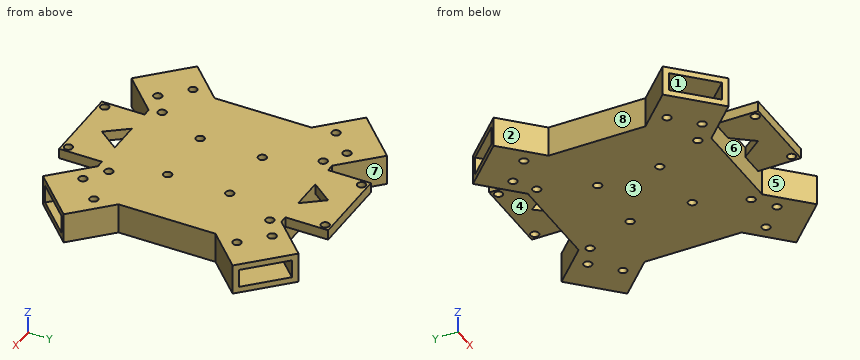
```python
from build123d import *

# Parameters (mm, degrees)
SKETCH1_W           = 90
SKETCH1_H           = 90
SKETCH1_R           = 2.05
BOSS_EXTRUDE1_DEPTH = 15
BOSS_EXTRUDE2_DEPTH = 15
SKETCH4_R           = 2.05
CUT_EXTRUDE1_DEPTH  = 15
SKETCH6_W           = 24
SKETCH6_H           = 9.009591428
CUT_EXTRUDE2_DEPTH  = 22
SKETCH9_W           = 24
SKETCH9_H           = 9
CUT_EXTRUDE3_DEPTH  = 22
SKETCH7_W           = 24
SKETCH7_H           = 9
CUT_EXTRUDE4_DEPTH  = 22
SKETCH8_W           = 24
SKETCH8_H           = 9
CUT_EXTRUDE5_DEPTH  = 22
SKETCH10_R          = 2.05
BOSS_EXTRUDE3_DEPTH = 5


with BuildPart() as part:
    # Sketch1 → Boss-Extrude1 (new body)
    with BuildSketch(Plane(origin=(0, 0, 0), x_dir=(0, 1, 0), z_dir=(0, 0, 1))):
        with Locations((-1.369565217, -20.064677945)):
            Rectangle(SKETCH1_W, SKETCH1_H)
        with Locations(Location((-40.369565217, 4.935322055, 0), (0, 0, 270))):
            Circle(SKETCH1_R, mode=Mode.SUBTRACT)
        with Locations(Location((-40.369565217, -45.064677945, 0), (0, 0, 270))):
            Circle(SKETCH1_R, mode=Mode.SUBTRACT)
        with Locations(Location((38.630434783, 4.935322055, 0), (0, 0, 270))):
            Circle(SKETCH1_R, mode=Mode.SUBTRACT)
        with Locations(Location((38.630434783, -45.064677945, 0), (0, 0, 270))):
            Circle(SKETCH1_R, mode=Mode.SUBTRACT)
        with Locations(Location((13.880434783, -4.814677945, 0), (0, 0, 270))):
            Circle(SKETCH1_R, mode=Mode.SUBTRACT)
        with Locations(Location((-16.619565217, -4.814677945, 0), (0, 0, 270))):
            Circle(SKETCH1_R, mode=Mode.SUBTRACT)
        with Locations(Location((13.880434783, -35.314677945, 0), (0, 0, 270))):
            Circle(SKETCH1_R, mode=Mode.SUBTRACT)
        with Locations(Location((-16.619565217, -35.314677945, 0), (0, 0, 270))):
            Circle(SKETCH1_R, mode=Mode.SUBTRACT)
    extrude(amount=BOSS_EXTRUDE1_DEPTH)

    # Sketch2 → Boss-Extrude2 (add)
    with BuildSketch(Plane.XY.offset(15)):
        Polygon((-21.399788149, 61.308104312), (-42.612991584, 40.094900877), (-24.935322055, 22.417231347), (-24.935322055, 43.630434783), (-3.722118619, 43.630434783), align=None)
        Polygon((-24.935322055, -25.156361782), (-42.612991584, -42.834031311), (-21.399788149, -64.047234747), (-3.722118619, -46.369565217), (-24.935322055, -46.369565217), align=None)
        Polygon((61.529144039, 61.308104312), (43.85147451, 43.630434783), (65.064677945, 43.630434783), (65.064677945, 22.417231347), (82.742347475, 40.094900877), align=None)
        Polygon((43.85147451, -46.369565217), (61.529144039, -64.047234747), (82.742347475, -42.834031311), (65.064677945, -25.156361782), (65.064677945, -46.369565217), align=None)
    extrude(amount=-BOSS_EXTRUDE2_DEPTH)

    # Sketch4 → Cut-Extrude1 (cut)
    with BuildSketch(Plane.XY.offset(15)):
        with Locations((-26.349535617, 33.730939846)):
            Circle(SKETCH4_R)
        with Locations((-15.035827118, 45.044648345)):
            Circle(SKETCH4_R)
        with Locations(Location((66.478891508, 33.730939846, 0), (0, 0, 180))):
            Circle(SKETCH4_R)
        with Locations(Location((55.165183009, 45.044648345, 0), (0, 0, 180))):
            Circle(SKETCH4_R)
        with Locations((66.478891508, -36.470070281)):
            Circle(SKETCH4_R)
        with Locations((55.165183009, -47.78377878)):
            Circle(SKETCH4_R)
        with Locations(Location((-15.035827118, -47.78377878, 0), (0, 0, 180))):
            Circle(SKETCH4_R)
        with Locations(Location((-26.349535617, -36.470070281, 0), (0, 0, 180))):
            Circle(SKETCH4_R)
    extrude(amount=-CUT_EXTRUDE1_DEPTH, mode=Mode.SUBTRACT)

    # Sketch6 → Cut-Extrude2 (cut)
    with BuildSketch(Plane(origin=(-41.35394623, 41.35394623, 0), x_dir=(-0.7071067811865476, -0.7071067811865476, 0), z_dir=(-0.7071067811865476, 0.7071067811865476, 0))):
        with Locations((-13.219440985, 7.504795714)):
            Rectangle(SKETCH6_W, SKETCH6_H)
    extrude(amount=-CUT_EXTRUDE2_DEPTH, mode=Mode.SUBTRACT)

    # Sketch9 → Cut-Extrude3 (cut)
    with BuildSketch(Plane(origin=(61.418624176, 61.418624176, 0), x_dir=(-0.7071067811865479, 0.7071067811865472, 0), z_dir=(0.7071067811865472, 0.7071067811865479, 0))):
        with Locations((-15.15629869, 7.5)):
            Rectangle(SKETCH9_W, SKETCH9_H)
    extrude(amount=-CUT_EXTRUDE3_DEPTH, mode=Mode.SUBTRACT)

    # Sketch7 → Cut-Extrude4 (cut)
    with BuildSketch(Plane(origin=(-42.723511448, -42.723511448, 0), x_dir=(0.7071067811865483, -0.7071067811865468, 0), z_dir=(-0.7071067811865468, -0.7071067811865483, 0))):
        with Locations((15.15629869, 7.5)):
            Rectangle(SKETCH7_W, SKETCH7_H)
    extrude(amount=-CUT_EXTRUDE4_DEPTH, mode=Mode.SUBTRACT)

    # Sketch8 → Cut-Extrude5 (cut)
    with BuildSketch(Plane(origin=(62.788189393, -62.788189393, 0), x_dir=(0.7071067811865461, 0.707106781186549, 0), z_dir=(0.707106781186549, -0.7071067811865461, 0))):
        with Locations((13.219440985, 7.5)):
            Rectangle(SKETCH8_W, SKETCH8_H)
    extrude(amount=-CUT_EXTRUDE5_DEPTH, mode=Mode.SUBTRACT)

    # Sketch10 → Boss-Extrude3 (add)
    # profile 1 of 2: a face of its own
    with BuildSketch(Plane.XY.offset(15)):
        Polygon((40.064677945, 64.630434783), (0.064677945, 64.630434783), (0.064677945, 43.630434783), (12.064677945, 43.630434783), (20.064677945, 54.130434783), (28.064677945, 43.630434783), (40.064677945, 43.630434783), align=None)
        with Locations((3.064677945, 61.630434783)):
            Circle(SKETCH10_R, mode=Mode.SUBTRACT)
        with Locations((37.064677945, 61.630434783)):
            Circle(SKETCH10_R, mode=Mode.SUBTRACT)
    # profile 2 of 2: a face of its own
    with BuildSketch(Plane.XY.offset(15)):
        Polygon((12.064677945, -46.369565217), (0.064677945, -46.369565217), (0.064677945, -67.369565217), (40.064677945, -67.369565217), (40.064677945, -46.369565217), (28.064677945, -46.369565217), (20.064677945, -56.869565217), align=None)
        with Locations((3.064677945, -64.369565217)):
            Circle(SKETCH10_R, mode=Mode.SUBTRACT)
        with Locations((37.064677945, -64.369565217)):
            Circle(SKETCH10_R, mode=Mode.SUBTRACT)
    extrude(amount=-BOSS_EXTRUDE3_DEPTH)


solid = part.part
```
CAD build for the part. Positions are in the model's coordinates, mm. Face numbers are marked on the shaded views. A direction names the side the tool comes from. Round coordinates to 2 decimals unless told otherwise and drop trailing zeros. Order: outer loops, then holes, each group sorted by start corner. A loop starts at its lowest first (then second) coordinate and runs counter-clockwise, first axis right, second up. Notation, with made-up numbers: (9, -25.75) -> (62, -25.75) arc R28 cw to (62, 1.25) -> close; hole circle Ø4 at (58.5, 72). An arc over 180 degrees is marked (long way). One line per question, with ' | ' between items.
Q1. Two-plate mould, pull along X, no slides. Class the marked faces 1, 2, 3 and 4: released by +X, released by -X, zero draft, split by the parting line, or undercut.
Completed:
face 1: undercut | face 2: released by -X | face 3: zero draft | face 4: undercut
Q2. Slice it at A-A (z = 1.5). Give the number of separate pieces and of enclosed holes in the cut face, then the cut area to 3 significant figures.
Completed:
separate pieces: 1 | enclosed holes: 16 | area: 9,990 mm^2
Q3. Drop flat-ended pins along their axis: pin 1 (2.5 mm diameter, centred on y = 58, z = 13.5, fed in from -X); pin 2 (1.5 mm diameter, centred on y = 58.5, z = 13, fed in from +X); pin 3 (6.5 mm diameter, centred on x = 35.31, y = -16.62, fed in from +Z); pin 4 (4 mm diameter, centred on y = -59.5, z = 12, fed in from +X). Give the stop position or say it passes through.
Completed:
pin 1: stops at x = -25.96 | pin 2: stops at x = 65.09 | pin 3: stops at z = 15 | pin 4: stops at x = 68.08
Q4. Slice it at B-B (y = 56.5). Write the cut outline in (x, z).
Completed:
outline: (-26.21, 0) -> (-16.59, 0) -> (-16.59, 15) -> (-26.21, 15) -> (-26.21, 12.01) -> (-20.83, 12.01) -> (-20.83, 3) -> (-26.21, 3) -> close; (0.06, 10) -> (40.06, 10) -> (40.06, 15) -> (0.06, 15) -> close; (56.72, 0) -> (66.34, 0) -> (66.34, 3) -> (60.96, 3) -> (60.96, 12) -> (66.34, 12) -> (66.34, 15) -> (56.72, 15) -> close
Q5. Slice it at C-C (x = 70.5). Write the cut outline in (y, z), then the cut area to 3 significant figures.
Completed:
outline: (-55.08, 0) -> (-30.59, 0) -> (-30.59, 15) -> (-55.08, 15) -> (-55.08, 12) -> (-34.83, 12) -> (-34.83, 3) -> (-55.08, 3) -> close; (27.85, 0) -> (52.34, 0) -> (52.34, 3) -> (32.1, 3) -> (32.1, 12) -> (52.34, 12) -> (52.34, 15) -> (27.85, 15) -> close | area: 370 mm^2
Q6. Slice it at D-D (x = 17.5). Write the cut outline in (y, z), then the cut area to 3 significant figures.
Completed:
outline: (-67.37, 10) -> (-53.5, 10) -> (-53.5, 15) -> (-67.37, 15) -> close; (-46.37, 0) -> (43.63, 0) -> (43.63, 15) -> (-46.37, 15) -> close; (50.76, 10) -> (64.63, 10) -> (64.63, 15) -> (50.76, 15) -> close | area: 1,490 mm^2
Q7. Which spindle directions (+Z, -Z, +X, -X, +Y, -Y) get a long thin tool onto all of the face, cutting with end or side? Do the marked faces 5, 6, 7 and 8. Say none if no direction does.
Completed:
face 5: +Z, -Z, -Y | face 6: -Z | face 7: +Z, -Z, +Y | face 8: +Z, -Z, -X
Q8. Probe probe 1 along Y at (x, z) = (-25, 2.25); probe 2 along Y at (x, z) = (-16.5, 8.25); probe 3 along Y at (x, z) = (-18, 7.5). List the from-to ranges inside material, lowest first.
Completed:
probe 1: y = -60.45 to -38.01, -34.93 to -25.22, 22.48 to 32.19, 35.27 to 57.71 | probe 2: y = -59.15 to -54.9, -37.83 to 35.1, 52.17 to 56.41 | probe 3: y = -60.65 to -56.4, -36.33 to 33.6, 53.67 to 57.91
